Autodesk Inventor part; units mm, degrees
ref_plane "YZ Plane" through (0, 0, 0) normal (1, 0, 0) x (0, 1, 0)
ref_plane "XZ Plane" through (0, 0, 0) normal (0, 1, 0) x (-1, 0, 0)
ref_plane "XY Plane" through (0, 0, 0) normal (0, 0, 1) x (1, 0, 0)
sketch "Sketch1" plane through (0, 0, 0) normal (0, 1, 0) x (-1, 0, 0)
  line L0 (14.0376, 28.5915) -> (4.0376, 28.5915)
  line L1 (4.0376, 28.5915) -> (4.0376, -31.4085)
  line L2 (4.0376, -31.4085) -> (14.0376, -31.4085)
  line L3 (14.0376, -31.4085) -> (14.0376, 28.5915)
  point P0 (0, 0)
  dimension "d0" = 60
  dimension "d1" = 10
extrude "Extrusion1" add sketch "Sketch1" along normal blind 5.2
sketch "Sketch2" plane through (0, 0, 0) normal (0, -1, 0) x (1, 0, 0)
  arc A0 (-14.0376, -26.4085) -> (-9.0376, -31.4085) centre (-9.0376, -26.4085) ccw
  arc A1 (-9.0376, 28.5915) -> (-14.0376, 23.5915) centre (-9.0376, 23.5915) ccw
  circle A2 centre (-9.0376, -26.4085) radius 1.5
  circle A3 centre (-9.0376, 23.5915) radius 1.5
  point P0 (0, 0)
fillet "Fillet1" radius 5 2 edges at (-14.0376, 2.6, -31.4085) (-14.0376, 2.6, 28.5915)
hole "Hole1" at (-9.0376, 0, -26.4085) at (-9.0376, 0, 23.5915) direction (0, 1, 0) diameter 3 end through all
sketch "Sketch3" plane through (0, 5.2, 0) normal (0, 1, 0) x (1, 0, 0)
  circle A0 centre (-2.0376, -12.5915) radius 7.9
  point P0 (0, 0)
extrude "Extrusion2" cut sketch "Sketch3" against normal blind 1.1
sketch "Sketch4" plane through (0, 4.1, 0) normal (0, 1, 0) x (1, 0, 0)
  circle A0 centre (-2.0376, -12.5915) radius 4.5
  circle A1 centre (24.4624, -12.0915) radius 6
  circle A2 centre (24.4624, 14.9085) radius 6
  circle A3 centre (-2.0376, 15.4085) radius 4.5
  circle A4 centre (30.9624, -22.5915) radius 3
  circle A5 centre (-9.0376, 26.4085) radius 3
  circle A6 centre (30.9624, 25.4085) radius 3
  circle A7 centre (-9.0376, -23.5915) radius 3
  arc A8 (4.9041, -26.2279) -> (6.8708, -28.5915) centre (6.8708, -26.5915) ccw
  line L0 (6.8708, -28.5915) -> (30.9624, -28.5915)
  arc A9 (30.9624, -28.5915) -> (35.9624, -23.5915) centre (30.9624, -23.5915) ccw
  line L1 (35.9624, -23.5915) -> (35.9624, 1.4085)
  line L2 (35.9624, 1.4085) -> (35.9624, 26.4085)
  arc A10 (35.9624, 26.4085) -> (30.9624, 31.4085) centre (30.9624, 26.4085) ccw
  line L3 (30.9624, 31.4085) -> (6.8708, 31.4085)
  arc A11 (6.8708, 31.4085) -> (4.9041, 29.0448) centre (6.8708, 29.4085) ccw
  arc A12 (-1.9792, 29.0448) -> (4.9041, 29.0448) centre (1.4624, 28.4085) ccw
  arc A13 (-1.9792, 29.0448) -> (-3.9459, 31.4085) centre (-3.9459, 29.4085) ccw
  line L4 (-3.9459, 31.4085) -> (-9.0376, 31.4085)
  arc A14 (-9.0376, 31.4085) -> (-14.0376, 26.4085) centre (-9.0376, 26.4085) ccw
  line L5 (-14.0376, 26.4085) -> (-14.0376, 1.4085)
  line L6 (-14.0376, 1.4085) -> (-14.0376, -23.5915)
  arc A15 (-14.0376, -23.5915) -> (-9.0376, -28.5915) centre (-9.0376, -23.5915) ccw
  line L7 (-9.0376, -28.5915) -> (-3.9459, -28.5915)
  arc A16 (-3.9459, -28.5915) -> (-1.9792, -26.2279) centre (-3.9459, -26.5915) ccw
  arc A17 (4.9041, -26.2279) -> (-1.9792, -26.2279) centre (1.4624, -25.5915) ccw
  circle A18 centre (-2.0376, -12.5915) radius 5.5
  circle A19 centre (-2.0376, -12.5915) radius 5.7
  point P0 (0, 0)
  dimension "d14" = 0.2
extrude "Extrusion3" cut sketch "Sketch4" against normal through all contours A0 | A18 | A19
properties part number "Carro XY_trava_A" material "ABS Plastic"
Model file for the job. Use its own axes, mm. A direction names the side the tool comes from. Round coordinates to 2 decimals unless told otherwise and drop trailing zeros. Write each loop counter-clockwise with the first axis right and the second up, starting at its lowest first coordinate (ties: lowest second). Pieces come first, ordered by that corner, then holes. Notation, with made-up numbers: (21.5, 5.5) - (46.5, 5.5) arc R31 cw to (46.5, 43.5) - close; hole circle Ø9 at (85, -20). An arc over 180 degrees is marked (long way). Use CSV: the item, a comma, the result in double quotes. Start each with the question number.
Item 1: Band-saw the part on B-B (z = 23). Write the cut outline in (x, y), and give its area (3 significant figures).
Item 2: Band-saw the part on C-C (x = -8.5). Write the cut outline in (y, z).
Item 3: Tool access for faces 5 (the face through (-7, 3, -31.408)), 6 (the face through (-9.936, 4.658, 12.446)): list every direction of +Z, -Z, +X, -X, +Y, -Y with a clear straight run to the whole face (end or side of a thin tool).
Item 4: Band-saw the part on D-D (x = -5.5). Write the cut outline in (y, z), and give its area (3 significant figures).
Item 5: Drill centre lines: L1, parallel to X at y = 3.6, z = -26.5; L2, parallel to Z at x = -8.5, y = 1.75; L3, parallel to Y at x = -5.75, z = 19.5. Where is each one in solid material? Low to high. Write a range as [from, to].
Item 6: Two-plate mould, pull along X, no slides. Class faces 1 (the face through (-12.6, 2.6, 27.1)), 2 (the face through (-4.038, 3, -12)), 3 (the face through (-8.12, 2.64, -25.22)), 4 (the face through (-8, 4.1, 12)): released by +X, released by -X, zero draft, split by the parting line, or undercut.
Item 7: Pin check, flat tip, straight feed: P1, Ø5, axis at x = -9.04, z = -26.41, coming from the +Y side. Stop position of the tip, or through.
Item 8: Band-saw the part on A-A (y = 2.3). Write the cut outline in (x, z), and give its area (3 significant figures).
Checked values:
1,outline,"(-14.04, 0) - (-10.42, 0) - (-10.42, 5.2) - (-14.04, 5.2) - close; (-7.66, 0) - (-4.04, 0) - (-4.04, 5.2) - (-7.66, 5.2) - close"
1,area,"37.7 mm²"
2,outline,"(0, -31.41) - (5.2, -31.41) - (5.2, -27.81) - (0, -27.81) - close; (0, -25.01) - (5.2, -25.01) - (5.2, 8.05) - (4.1, 8.05) - (4.1, 17.14) - (5.2, 17.14) - (5.2, 22.19) - (0, 22.19) - close; (0, 24.99) - (5.2, 24.99) - (5.2, 28.59) - (0, 28.59) - close"
3,face 5,"-Z, +X, -X, +Y, -Y"
3,face 6,"+X, +Y"
4,outline,"(0, -31.41) - (5.2, -31.41) - (5.2, 5.49) - (4.1, 5.49) - (4.1, 8.06) - (0, 8.06) - close; (0, 17.12) - (4.1, 17.12) - (4.1, 19.69) - (5.2, 19.69) - (5.2, 28.59) - (0, 28.59) - close"
4,area,"259 mm²"
5,L1,"x = [-14.04, -10.53], [-7.54, -4.04]"
5,L2,"z = [-31.41, -27.81], [-25.01, 22.19], [24.99, 28.59]"
5,L3,"y = [0, 4.1]"
6,face 1,"released by -X"
6,face 2,"released by +X"
6,face 3,"undercut"
6,face 4,"zero draft"
7,P1,"stops at y = 5.2"
8,outline,"(-14.04, -26.41) arc R5 ccw to (-9.04, -31.41) - (-4.04, -31.41) - (-4.04, 7.25) arc R5.7 cw to (-4.04, 17.93) - (-4.04, 28.59) - (-9.04, 28.59) arc R5 ccw to (-14.04, 23.59) - close; hole circle Ø3 at (-9.04, -26.41); hole circle Ø3 at (-9.04, 23.59)"
8,area,"546 mm²"
